from build123d import *

# Parameters (mm, degrees)
SKETCH_1_R          = 2.25
SKETCH_1_R_2        = 13
EXTRUDE_1_DEPTH     = 15
EXTRUDE_START       = -15
SKETCH_2_R          = 13
EXTRUDE_2_DEPTH     = 15
SKETCH_3_R          = 15.5
SKETCH_3_R_2        = 13
CUT_EXTRUDE_1_DEPTH = 10
FILLET_2_DEPTH      = 15
SHELL_1_T           = -2


with BuildPart() as part:
    # Sketch 1 → Extrude 1 (new body)
    with BuildSketch(Plane.XY):
        with BuildLine():
            Line((-20.509328188, 29.527748201), (-45.909328188, 29.527748201))
            Line((-45.909328188, 29.527748201), (-45.909328188, 9.527748201))
            Line((-45.909328188, 9.527748201), (-41.345035516, 9.527748201))
            ThreePointArc((-41.345035516, 9.527748201), (-42.891279982, -2.208471939), (-38.288719604, -13.114716624))
            Line((-38.288719604, -13.114716624), (-40.944647776, -16.120109029))
            ThreePointArc((-40.944647776, -16.120109029), (-40.661470992, -20.707571357), (-36.07400866, -20.424394637))
            Line((-36.07400866, -20.424394637), (-33.582654856, -17.603814511))
            ThreePointArc((-33.582654856, -17.603814511), (-27.370227174, -20.704922292), (-20.509328188, -21.772251799))
            ThreePointArc((-20.509328188, -21.772251799), (2.605029944, -7.24200666), (-0.468314839, 19.886504679))
            Line((-0.468314839, 19.886504679), (2.117446855, 22.813968467))
            ThreePointArc((2.117446855, 22.813968467), (1.525885658, 27.261599934), (-2.944647715, 26.87989104))
            Line((-2.944647715, 26.87989104), (-5.1306618, 24.406243523))
            ThreePointArc((-5.1306618, 24.406243523), (-12.404804913, 28.213713407), (-20.509328188, 29.527748201))
        make_face()
        with Locations((-38.509328188, -18.272251799)):
            Circle(SKETCH_1_R, mode=Mode.SUBTRACT)
        with Locations((-0.509328188, 24.727748201)):
            Circle(SKETCH_1_R, mode=Mode.SUBTRACT)
        with Locations((-20.509328188, 1.727748201)):
            Circle(SKETCH_1_R_2, mode=Mode.SUBTRACT)
    extrude(amount=EXTRUDE_1_DEPTH)

    # Sketch 2 → Extrude 2 (add)
    with BuildSketch(Plane.XY.offset(15).offset(EXTRUDE_START)):
        with Locations((-20.509328188, 1.727748201)):
            Circle(SKETCH_2_R)
    extrude(amount=EXTRUDE_2_DEPTH)

    # Sketch 3 → Cut-Extrude 1 (cut)
    with BuildSketch(Plane.XY.offset(15)):
        with Locations((-20.509328188, 1.727748201)):
            Circle(SKETCH_3_R)
        with Locations((-20.509328188, 1.727748201)):
            Circle(SKETCH_3_R_2, mode=Mode.SUBTRACT)
    extrude(amount=-CUT_EXTRUDE_1_DEPTH, mode=Mode.SUBTRACT)

    # Fillet 2: read off the stored shape, not the designer's step
    # Fillet 2 outline → Fillet 2 (add)
    with BuildSketch(Plane.XY):
        with BuildLine():
            add(Edge.make_bspline(
                [(-6.538335188, 25.388997691), (-5.092197369, 24.449769063), (-3.950320838, 25.741892507)],
                knots=[0, 0, 0, 1, 1, 1], degree=2, weights=[1, 0.757365787, 1]))
            ThreePointArc((-6.538335188, 25.388997691), (-5.826274078, 24.909401062), (-5.1306618, 24.406243523))
            Line((-5.1306618, 24.406243523), (-3.950320838, 25.741892507))
        make_face()
        with BuildLine():
            add(Edge.make_bspline(
                [(-32.195062511, -18.514056777), (-33.623677266, -17.650257933), (-34.728876524, -18.901506574)],
                knots=[0, 0, 0, 1, 1, 1], degree=2, weights=[1, 0.767694161, 1]))
            ThreePointArc((-32.195062511, -18.514056777), (-32.897221897, -18.071684701), (-33.582654856, -17.603814511))
            Line((-33.582654856, -17.603814511), (-34.728876524, -18.901506574))
        make_face()
        with BuildLine():
            add(Edge.make_bspline(
                [(0.60935837, 21.106589771), (-0.435699032, 19.923430585), (0.472348447, 18.632128758)],
                knots=[0, 0, 0, 1, 1, 1], degree=2, weights=[1, 0.784947091, 1]))
            Line((0.60935837, 21.106589771), (-0.468314839, 19.886504679))
            ThreePointArc((-0.468314839, 19.886504679), (0.011603519, 19.266505848), (0.472348447, 18.632128758))
        make_face()
        with BuildLine():
            add(Edge.make_bspline(
                [(-39.352533344, -14.318505855), (-38.32459871, -13.155316664), (-39.196367828, -11.87091902)],
                knots=[0, 0, 0, 1, 1, 1], degree=2, weights=[1, 0.789973537, 1]))
            Line((-39.352533344, -14.318505855), (-38.288719604, -13.114716624))
            ThreePointArc((-38.288719604, -13.114716624), (-38.7531465, -12.500555092), (-39.196367828, -11.87091902))
        make_face()
    extrude(amount=FILLET_2_DEPTH)

    # Shell 1
    shell_1_openings = [part.faces().sort_by_distance(p)[0] for p in [
        (-45.909328188, 19.527748201, 7.5),
    ]]
    offset(amount=SHELL_1_T, openings=shell_1_openings, kind=Kind.INTERSECTION)


solid = part.part
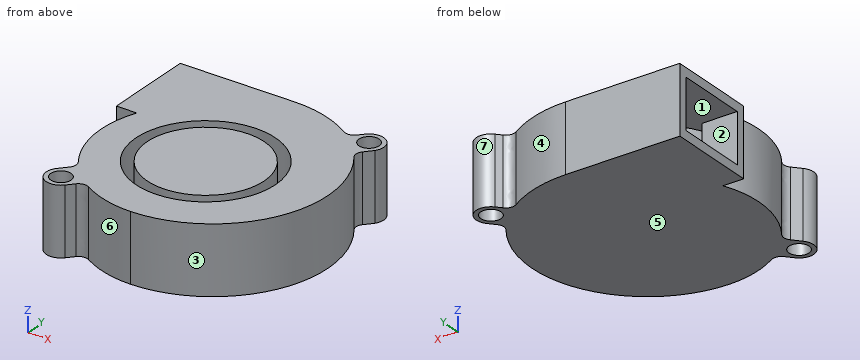
Read the model definition and answer for the solid it produces. Units are mm, in the model's axes. Face numbers are marked on the shaded views. A direction names the side the tool comes from. Give positions to 0.01 mm unless a question says otherwise; leave off trailing zeros. Loops run counter-clockwise (first coordinate to the right, second up) from the corner with the lowest first, then second, coordinate; pieces in that order, holes last. Notation, with made-up numbers: (-1.5, 82) -> (18.5, 82) arc R12 ccw to (18.5, 99) -> close; hole circle Ø4 at (77, 46.25). An arc over 180 degrees is marked (long way). Answer as CSV lines item,"result".
Item 1: Find section C-C on z = 11.75. State how many separate pieces and enclosed holes the cut face has, plus the area to 3 significant figures.
Returned:
separate pieces,"3"
enclosed holes,"4"
area,"699 mm²"
Item 2: Find section B-B on y = 3.5. Give the vertices of the cut face in (x, z), plus the area to 3 significant figures.
Returned:
outline,"(-42.93, 0) -> (5.14, 0) -> (5.14, 15) -> (-5.11, 15) -> (-5.11, 5) -> (-7.63, 5) -> (-7.63, 15) -> (-33.39, 15) -> (-33.39, 5) -> (-35.91, 5) -> (-35.91, 15) -> (-42.93, 15) -> close; hole (-40.92, 2) -> (3.14, 2) -> (3.14, 13) -> (-3.1, 13) -> (-3.1, 3) -> (-9.65, 3) -> (-9.65, 13) -> (-31.37, 13) -> (-31.37, 3) -> (-37.92, 3) -> (-37.92, 13) -> (-40.92, 13) -> close"
area,"317 mm²"
Item 3: Find section A-A on x = -12.5. Give the vertices of the cut face in (y, z).
Returned:
outline,"(-20.49, 0) -> (28.25, 0) -> (28.25, 15) -> (15, 15) -> (15, 5) -> (11.97, 5) -> (11.97, 15) -> (-8.51, 15) -> (-8.51, 5) -> (-11.54, 5) -> (-11.54, 15) -> (-20.49, 15) -> close; hole (-18.37, 2) -> (26.13, 2) -> (26.13, 13) -> (17.29, 13) -> (17.29, 3) -> (9.27, 3) -> (9.27, 13) -> (-5.81, 13) -> (-5.81, 3) -> (-13.83, 3) -> (-13.83, 13) -> (-18.37, 13) -> close"
Item 4: Determine the mould class of the marked faces 4, 5, 6 and 7 for opening direction Y: +Y half, -Y half, draft (parallel to the pull), parting line (faces both ways), or undercut.
Returned:
face 4,"+Y half"
face 5,"draft"
face 6,"-Y half"
face 7,"undercut"
Item 5: Each of these flat-tipped pins is pushed along its axis until it touches: pin 1 (1.5 mm diameter, centred on y = -1.5, z = 4, fed in from -X); pin 2 (1 mm diameter, centred on x = -14.5, z = 6, fed in from -Y); pin 3 (5 mm diameter, centred on x = -3.5, z = 6.5, fed in from -Y). Where does it stop, or does it pass through?
Returned:
pin 1,"stops at x = -43.04"
pin 2,"stops at y = -21.17"
pin 3,"stops at y = -17.27"
Item 6: Find section D-D on y = 15.5. Give the vertices of the cut face in (x, z).
Returned:
outline,"(-45.91, 0) -> (2.36, 0) -> (2.36, 15) -> (-13.4, 15) -> (-13.4, 5) -> (-27.62, 5) -> (-27.62, 15) -> (-45.91, 15) -> (-45.91, 13) -> (-31.31, 13) -> (-31.31, 3) -> (-9.71, 3) -> (-9.71, 13) -> (0.09, 13) -> (0.09, 2) -> (-45.91, 2) -> close"
Item 7: Consider line 1 (Z direction, x = -13.5, y = -18); line 2 (Y direction, x = -34, z = 10.25); line 3 (Y direction, x = -2.5, z = 4). Determine where each line is inside the solid, lowest interval first. Write a range as [from, to].
Returned:
line 1,"z = [0, 2], [13, 15]"
line 2,"y = [-18.38, -16.3], [-9.42, -5.9], [9.36, 12.87], [27.53, 29.53]"
line 3,"y = [-14.39, -11.45], [20.97, 23.68], [25.78, 27.3]"
Item 8: For the marked faces 1, 2 and 3, determine the directions among +Z, -Z, +X, -X, +Y, -Y from which every point of the face is accessible in a straight line to the end or side of a thin tool.
Returned:
face 1,"none"
face 2,"-X"
face 3,"+Z, -Z, +X"
